Input: part model. Units: mm. Frame: model coordinates. Face numbers are marked on the shaded views. A direction names the side the tool comes from. Round coordinates to 2 decimals unless told otherwise and drop trailing zeros. Order: outer loops, then holes, each group sorted by start corner. A loop starts at its lowest first (then second) coordinate and runs counter-clockwise, first axis right, second up. Notation, with made-up numbers: M -40,-1.5 L -11,-1.5 A23 cw -11,9.5 Z; hole C 51,15.5 d5. An arc over 180 degrees is marked long. One line per question, with ' | ' between items.
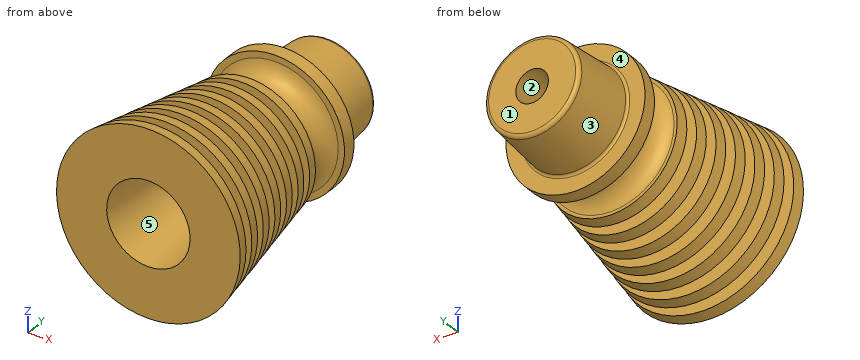
```python
from build123d import *

# Parameters (mm, degrees)
SKETCH5_R          = 1.6383
CUT_EXTRUDE1_DEPTH = 27.4668
FILLET1_R          = 0.381
FILLET2_R          = 0.254


with BuildPart() as part:
    # Sketch1 → Revolve1 (revolve)
    with BuildSketch(Plane.XY, mode=Mode.PRIVATE) as revolve1_sk:
        Polygon((4.571997254, 14.859), (6.235697254, 0), (4.191, 0), (2.5273, 14.859), align=None)
    revolve(revolve1_sk.sketch.rotate(Axis((0, 0, 0), (0, 1, 0)), 90), axis=Axis((0, 0, 0), (0, 1, 0)))  # turned: the seam where the file's is

    # Sketch2 → Revolve2 (revolve)
    with BuildSketch(Plane.XY, mode=Mode.PRIVATE) as revolve2_sk:
        Polygon((6.235697254, 0), (9.2329, 0), (9.035561538, 1.143), (6.107720331, 1.143), align=None)
        Polygon((4.571997254, 14.859), (4.699974177, 13.716), (6.864838462, 13.716), (6.6675, 14.859), align=None)
        Polygon((5.979743408, 2.286), (8.838223077, 2.286), (8.640884615, 3.429), (5.851766485, 3.429), align=None)
        Polygon((5.723789562, 4.572), (8.443546154, 4.572), (8.246207692, 5.715), (5.595812639, 5.715), align=None)
        Polygon((5.467835716, 6.858), (8.048869231, 6.858), (7.851530769, 8.001), (5.339858793, 8.001), align=None)
        Polygon((5.21188187, 9.144), (7.654192308, 9.144), (7.456853846, 10.287), (5.083904947, 10.287), align=None)
        Polygon((4.955928023, 11.43), (7.259515385, 11.43), (7.062176923, 12.573), (4.8279511, 12.573), align=None)
    revolve(revolve2_sk.sketch.rotate(Axis((0, 0, 0), (0, 1, 0)), 90), axis=Axis((0, 0, 0), (0, 1, 0)))  # turned: the seam where the file's is

    # Sketch3 → Revolve3 (revolve)
    with BuildSketch(Plane.XY, mode=Mode.PRIVATE) as revolve3_sk:
        with BuildLine():
            Line((6.35, 14.859), (0, 14.859))
            Line((0, 14.859), (0, 20.066))
            Line((0, 20.066), (6.985, 20.066))
            Line((6.985, 20.066), (6.985, 18.669))
            Line((6.985, 18.669), (6.35, 18.669))
            ThreePointArc((6.35, 18.669), (4.6863, 16.764), (6.35, 14.859))
        make_face()
    revolve(revolve3_sk.sketch.rotate(Axis((0, 0, 0), (0, 1, 0)), 90), axis=Axis((0, 0, 0), (0, 1, 0)))  # turned: the seam where the file's is

    # Sketch4 → Revolve4 (revolve)
    with BuildSketch(Plane.XY, mode=Mode.PRIVATE) as revolve4_sk:
        Polygon((5.2197, 20.066), (0, 20.066), (0, 26.4668), (4.733451381, 26.4668), align=None)
    revolve(revolve4_sk.sketch.rotate(Axis((0, 0, 0), (0, 1, 0)), 90), axis=Axis((0, 0, 0), (0, 1, 0)))  # turned: the seam where the file's is

    # Sketch5 → Cut-Extrude1 (cut, through all)
    with BuildSketch(Plane(origin=(0, 26.4668, 0), x_dir=(1, 0, 0), z_dir=(0, 1, 0))):
        with Locations(Location((0, 0, 0), (0, 0, 270))):  # turned: the seam where the file's is
            Circle(SKETCH5_R)
    extrude(amount=-CUT_EXTRUDE1_DEPTH, mode=Mode.SUBTRACT)

    # Fillet1
    fillet1_edges = [part.edges().sort_by_distance(p)[0] for p in [
        (0, 26.4668, 4.733451381),
    ]]
    fillet(fillet1_edges, radius=FILLET1_R)

    # Fillet2
    fillet2_edges = [part.edges().sort_by_distance(p)[0] for p in [
        (0, 20.066, 5.2197),
    ]]
    fillet(fillet2_edges, radius=FILLET2_R)


solid = part.part
```
Item 1: Access query for the marked faces 4 and 5. Directions: +Z, -Z, +X, -X, +Y, -Y. A direction counts if a zero-diameter tool reaches every point of the face in a straight line with its end or side. Return the directions, or none.
Report:
face 4: +Y | face 5: -Y
Item 2: First-contact query: pin 1 (10 mm diameter, centred on x = 4, y = 17, fed in from -Z) (3 decimals); pin 2 (8 mm diameter, centred on x = 5.5, z = -3.5, fed in from +Y); pin 3 (2 mm diameter, centred on y = 20.5, z = -5.5, fed in from -X); pin 4 (4 mm diameter, centred on x = 0, z = 0, fed in from -Y). Flat tips, straight axial feed; report the tip coordinate or a pass-through.
Report:
pin 1: z = -6.985 | pin 2: y = 26.47 | pin 3: x = -5.26 | pin 4: y = 14.86
Item 3: Mould query, pull axis Z, two halves, no side actions, for the marked faces 1, 2 and 3. Classes: +Z half, -Z half, draft (parallel to the pull), parting line (faces both ways), or undercut.
Report:
face 1: draft | face 2: undercut | face 3: parting line
Item 4: Line query: line 1 along Y through (x, z) = (-0.75, 1.5); line 2 along Y through (x, z) = (4, 4) (3 decimals); line 3 along X through (y, z) = (23, 0). Output: solid intervals per line, ascending. Write a range as from..to.
Report:
line 1: 14.86..26.47 | line 2: 0..5.715, 6.858..8.001, 9.144..10.287, 11.43..12.573, 13.716..15.094, 18.434..20.066 | line 3: -5..-1.64, 1.64..5
Item 5: Section query A-A, the plane y = 24.75. Return loops of the section in (x, z), plus the area to 3 significant figures.
Report:
outline: C 0,0 d9.73; hole C 0,0 d3.28 | area: 65.9 mm²
